```python
from build123d import *

# Parameters (mm, degrees)
F1_DEPTH  = 80
F3_DEPTH  = 40
F5_R      = 31.25
F6_DEPTH  = 50.2
F7_ANGLE  = 90
F9_DEPTH  = 4
F10_DEPTH = 4
F12_DEPTH = 67.8795645455


with BuildPart() as f1:
    # F0 (on Front) → F1 (new body)
    with BuildSketch(Plane.XZ):
        with BuildLine():
            ThreePointArc((30.4294233557, -17.2930678088), (33.8380689272, -8.9434384481), (35, 0))
            ThreePointArc((35, 0), (0, 35), (-35, 0))
            ThreePointArc((-35, 0), (-33.8380689272, -8.9434384481), (-30.4294233557, -17.2930678088))
            ThreePointArc((-30.4294233557, -17.2930678088), (-27.1770371159, -17.1981120299), (-25.5228132327, -20))
            ThreePointArc((-25.5228132327, -20), (-25.8531904298, -21.4160737865), (-26.7761038382, -22.5397485178))
            ThreePointArc((-26.7761038382, -22.5397485178), (0, -35), (26.7761038382, -22.5397485178))
            ThreePointArc((26.7761038382, -22.5397485178), (26.0967274514, -18.1714285714), (30.4294233557, -17.2930678088))
        make_face()
        with BuildLine():
            Line((35, -40), (35, 0))
            ThreePointArc((35, 0), (33.8380689272, -8.9434384481), (30.4294233557, -17.2930678088))
            ThreePointArc((30.4294233557, -17.2930678088), (31.5247012028, -18.4542238832), (31.9228132327, -20))
            ThreePointArc((31.9228132327, -20), (30.1388870192, -22.8696228029), (26.7761038382, -22.5397485178))
            ThreePointArc((26.7761038382, -22.5397485178), (0, -35), (-26.7761038382, -22.5397485178))
            ThreePointArc((-26.7761038382, -22.5397485178), (-31.348899014, -21.8285714286), (-30.4294233557, -17.2930678088))
            ThreePointArc((-30.4294233557, -17.2930678088), (-33.8380689272, -8.9434384481), (-35, 0))
            Line((-35, 0), (-35, -40))
            Line((-35, -40), (35, -40))
        make_face()
    extrude(amount=F1_DEPTH)

    # F2 (on face) → F3 (cut)
    with BuildSketch(Plane.XZ.offset(80)):
        with BuildLine():
            ThreePointArc((-31.25, 0), (0, -31.25), (31.25, 0))
            ThreePointArc((31.25, 0), (0, 31.25), (-31.25, 0))
        make_face()
        with BuildLine():
            ThreePointArc((-31.25, 0), (0, 31.25), (31.25, 0))
            Line((31.25, 0), (35, 0))
            ThreePointArc((35, 0), (0, 35), (-35, 0))
            Line((-35, 0), (-31.25, 0))
        make_face()
    extrude(amount=-F3_DEPTH, mode=Mode.SUBTRACT)

    # F5 (on offset) → F6 (cut)
    with BuildSketch(Plane.XY):
        with Locations((0, -40)):
            Circle(F5_R)
    extrude(amount=F6_DEPTH, mode=Mode.SUBTRACT)

    # F6_face (on face) → F7 (revolve, cut)
    with BuildSketch(Plane(origin=(0, -26.7370880757, 0), x_dir=(1, 0, 0), z_dir=(0, 0, 1))):
        with BuildLine():
            Line((-31.25, -13.2629119243), (31.25, -13.2629119243))
            ThreePointArc((31.25, -13.2629119243), (0, 17.9870880757), (-31.25, -13.2629119243))
        make_face()
    revolve(axis=Axis((0, -40, 0), (-1, 0, 0)), revolution_arc=F7_ANGLE, mode=Mode.SUBTRACT)

    # F8 (on face) → F9 (cut)
    with BuildSketch(Plane(origin=(0, 0, 0), x_dir=(-1, 0, 0), z_dir=(0, 1, 0))):
        Polygon((-32.8785644455, 18), (-32.8785644455, 12), (0, 12), (32.8785644455, 12), (32.8785644455, 18), align=None)
    extrude(amount=-F9_DEPTH, mode=Mode.SUBTRACT)

    # F8 (on face) → F10 (join)
    with BuildSketch(Plane(origin=(0, 0, 0), x_dir=(-1, 0, 0), z_dir=(0, 1, 0))):
        Polygon((-32.8785644455, 18), (-32.8785644455, 12), (0, 12), (32.8785644455, 12), (32.8785644455, 18), align=None)
    extrude(amount=-F10_DEPTH)

    # F11 (on face) → F12 (cut, through all)
    with BuildSketch(Plane.YZ.offset(32.8785644455)):
        with BuildLine():
            ThreePointArc((-4, 18), (-7, 15), (-4, 12))
            Line((-4, 12), (0, 12))
            Line((0, 12), (0, 18))
            Line((0, 18), (-4, 18))
        make_face()
    extrude(amount=-F12_DEPTH, mode=Mode.SUBTRACT)


solid = f1.part
```
Part model, mm, in its own coordinate system. A direction names the side the tool comes from. Round coordinates to 2 decimals unless told otherwise and drop trailing zeros. Loops run counter-clockwise (first coordinate to the right, second up) from the corner with the lowest first, then second, coordinate; pieces in that order, holes last. Notation, with made-up numbers: (-10.75, -29) -> (34.25, -29) arc R14 ccw to (34.25, -8) -> close; hole circle Ø10 at (19.5, -19.75). An arc over 180 degrees is marked (long way). Use CSV: the item, a comma, the result in double quotes. Start each with the question number.
1) Pull direction X, two halves, no side cores. Call faces 1 (the flat face through (-35, -39, -20)), 2 (the cylindrical face through (0, -7, 15)), 3 (the cylindrical face through (-0.687, -60.28, -31.242)), 4 (the cylindrical face through (0.687, -8.758, 13.367)): +X half, -X half, draft (parallel to the pull), parting line (faces both ways), or undercut.
2) Cut at D-D, the plane y = -30.5. Write the cut outline in (x, z), plus the area to 3 significant figures.
3) Which spindle directions (+Z, -Z, +X, -X, +Y, -Y) get a long thin tool onto all of the face, cutting with end or side? Do faces 5 (the flat face through (0, -80, -33)), 6 (the flat face through (0, -2, 12)), 7 (the flat face through (33, -40, 6)). Say none if no direction does.
4) Drop flat-ended pins along their axis: P1, Ø2, axis at x = 10, y = -2.5, coming from the +Z side; P2, Ø10, axis at x = 22, y = -43.5, coming from the +Z side; P3, Ø3, axis at x = 16.5, z = -18.5, coming from the +Y side; P4, Ø1.9, axis at x = -32.5, y = -58, coming from the +Z side. Give the stop position or say it passes through.
5) Cut at B-B, the plane x = 0. Write the cut outline in (y, z).
6) Wall check: L1, parallel to X at y = -53, z = -19.5; L2, parallel to Z at x = 1, y = -49; L3, parallel to X at y = -33, z = 15.5. Give the ranges that are in metal, low to high. Write a range as [from, to].
7) Cut at A-A, the plane y = -68. Write the cut outline in (x, z).
8) Cut at C-C, the plane z = -13.5. Write the cut outline in (x, y), plus the area to 3 significant figures.
Determined:
1,face 1,"-X half"
1,face 2,"draft"
1,face 3,"undercut"
1,face 4,"undercut"
2,outline,"(-35, -40) -> (35, -40) -> (35, 0) arc R35 ccw to (29.77, 18.4) -> (29.77, 0) arc R29.77 cw to (-29.77, 0) -> (-29.77, 18.4) arc R35 ccw to (-35, 0) -> close; hole circle Ø6.4 at (-28.72, -20); hole circle Ø6.4 at (28.72, -20)"
2,area,"1,470 mm2"
3,face 5,"+Z, -Z, +X, -X, -Y"
3,face 6,"+X, -X, +Y"
3,face 7,"+Z, +X, -X, -Y"
4,P1,"stops at z = 33.82"
4,P2,"stops at z = -15.73"
4,P3,"stops at y = 0"
4,P4,"stops at z = 0"
5,outline,"(-80, -40) -> (0, -40) -> (0, 12) -> (-4, 12) arc R3 cw to (-4, 18) -> (0, 18) -> (0, 35) -> (-8.75, 35) -> (-8.75, 0) arc R31.25 cw to (-40, -31.25) -> (-80, -31.25) -> close"
6,L1,"x = [-35, -31.88], [-25.56, -24.42], [24.42, 25.56], [31.88, 35]"
6,L2,"z = [-40, -31.23]"
6,L3,"x = [-31.38, -30.46], [30.46, 31.38]"
7,outline,"(-35, -40) -> (35, -40) -> (35, 0) -> (31.25, 0) arc R31.25 cw to (-31.25, 0) -> (-35, 0) -> close; hole circle Ø6.4 at (-28.72, -20); hole circle Ø6.4 at (28.72, -20)"
8,outline,"(-35, -80) -> (-28.18, -80) -> (-28.18, -40) arc R28.18 cw to (28.18, -40) -> (28.18, -80) -> (35, -80) -> (35, 0) -> (-35, 0) -> close"
8,area,"2,100 mm2"
